The listing builds one solid part. Answer for the finished solid, in the listing's coordinates (mm). Face numbers are marked on the shaded views. Give positions to 0.01 mm unless a question says otherwise; leave off trailing zeros. Write each loop counter-clockwise with the first axis right and the second up, starting at its lowest first coordinate (ties: lowest second). Pieces come first, ordered by that corner, then holes. Notation, with made-up numbers: M 68,64 L 125,64 A26 ccw 125,97 Z; hole C -12,51 d5. An arc over 180 degrees is marked long. Return JSON: item names as keys, results as strings.
from build123d import *

# Parameters (mm, degrees)
SKETCH_1_W          = 100
SKETCH_1_H          = 200
SKETCH_1_R          = 40
EXTRUDE_1_DEPTH     = 10
SKETCH_2_W          = 100
SKETCH_2_H          = 250
EXTRUDE_2_DEPTH     = 10
SKETCH_3_R          = 40
CUT_EXTRUDE_1_DEPTH = 136


with BuildPart() as part:
    # 草图1 → 凸台-拉伸1 (new body)
    with BuildSketch(Plane.XY):
        Rectangle(SKETCH_1_W, SKETCH_1_H)
        with Locations((0, 50)):
            Circle(SKETCH_1_R, mode=Mode.SUBTRACT)
        with Locations(Location((0, -50, 0), (0, 0, 180))):
            Circle(SKETCH_1_R, mode=Mode.SUBTRACT)
    extrude(amount=EXTRUDE_1_DEPTH)

    # 草图2 → 凸台-拉伸2 (add)
    with BuildSketch(Plane.XY.offset(10)):
        Rectangle(SKETCH_2_W, SKETCH_2_H)
    extrude(amount=EXTRUDE_2_DEPTH)

    # 草图3 → 切除-拉伸1 (cut, through all)
    with BuildSketch(Plane(origin=(0, 0, 10), x_dir=(-1, 0, 0), z_dir=(0, 0, -1))):
        with Locations((0, 50)):
            Circle(SKETCH_3_R)
        with Locations((0, -50)):
            Circle(SKETCH_3_R)
    extrude(amount=-CUT_EXTRUDE_1_DEPTH, mode=Mode.SUBTRACT)


solid = part.part
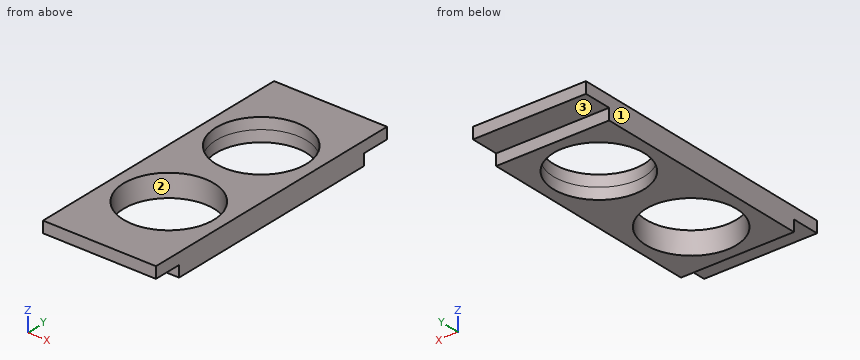
Item 1: A cutting plane is placed at D-D, the plane y = -87. Write down the section's boundary in (x, z), plus the area to 3 significant figures.
Geometry results:
{"outline": "M -50,0 L -15.2,0 L -15.2,20 L -50,20 Z; M 15.2,0 L 50,0 L 50,20 L 15.2,20 Z", "area": "1,390 mm2"}
Item 2: A cutting plane is placed at A-A, the plane y = 50. Write down the section's boundary in (x, z), plus the area to 3 significant figures.
Geometry results:
{"outline": "M -50,0 L -40,0 L -40,20 L -50,20 Z; M 40,0 L 50,0 L 50,20 L 40,20 Z", "area": "400 mm2"}
Item 3: A cutting plane is placed at B-B, the plane x = 0. Write down the section's boundary in (y, z).
Geometry results:
{"outline": "M -125,10 L -100,10 L -100,0 L -90,0 L -90,20 L -125,20 Z; M -10,0 L 10,0 L 10,20 L -10,20 Z; M 90,0 L 100,0 L 100,10 L 125,10 L 125,20 L 90,20 Z"}
Item 4: Determine the mould class of the marked faces 1, 2 and 3 for opening direction X: +X half, -X half, draft (parallel to the pull), parting line (faces both ways), or undercut.
Geometry results:
{"face 1": "-X half", "face 2": "undercut", "face 3": "draft"}
Item 5: A cutting plane is placed at C-C, the plane z = 15.25. Write down the section's boundary in (x, y).
Geometry results:
{"outline": "M -50,-125 L 50,-125 L 50,125 L -50,125 Z; hole C 0,-50 d80; hole C 0,50 d80"}
Item 6: Find the intervals of material crossed by line 1 (Y direction, x = 0, z = 15.75); line 2 (Y direction, x = 0, z = 5.75); line 3 (X direction, y = -50, z = 6), in increasing order.
Geometry results:
{"line 1": "y = -125 to -90, -10 to 10, 90 to 125", "line 2": "y = -100 to -90, -10 to 10, 90 to 100", "line 3": "x = -50 to -40, 40 to 50"}
Item 7: Given pin 1 Ø1 at (x, z) = (-25.5, 2.5) entering from -Y; pin 2 Ø4 at (x, z) = (35.5, 4.5) entering from +Y; pin 3 Ø7.5 at (x, y) = (-3.5, -112.5) entering from -Z, each flat-ended and moving along its own axis, determine where each tip first touches the part or whether it passes through.
Geometry results:
{"pin 1": "stops at y = -100", "pin 2": "stops at y = 100", "pin 3": "stops at z = 10"}
